from build123d import *

# Parameters (mm, degrees)
CIRPATTERN1_COUNT           = 8
LPATTERN1_START             = -24.818843944
LPATTERN1_OUTLINE_R         = 41.275
LPATTERN1_OUTLINE_R_2       = 38.453474767
LPATTERN1_DEPTH             = 5.187687888
LPATTERN1_START_2           = -12.118843944
LPATTERN1_2_OUTLINE_R       = 41.275
LPATTERN1_2_OUTLINE_R_2     = 38.453474767
LPATTERN1_2_DEPTH           = 5.187687888
SKETCH15_R                  = 53.975
SKETCH15_R_2                = 19.05
BOSS_EXTRUDE1_DEPTH         = 5.08
Q_0_332_DIAMETER_HOLE1_D    = 8.4328
F_1_4_0_25_DIAMETER_HOLE1_D = 6.35
CIRPATTERN2_COUNT           = 6


# Read off the part's stored shape, not the designer's step: LPattern1
with BuildPart() as part:
    # Sketch1 → Revolve1 (revolve)
    with BuildSketch(Plane.XY, mode=Mode.PRIVATE) as revolve1_sk:
        Polygon((-41.275, -40.64), (-41.275, 0), (-34.925, 0), (-34.925, -25.4), (-13.91158, -25.4), (-13.91158, -74.93), (-8.90651, -74.93), (-8.90651, -88.392), (-19.05, -88.392), (-19.05, -40.64), align=None)
    revolve(revolve1_sk.sketch.rotate(Axis((0, 0, 0), (0, 1, 0)), 270), axis=Axis((0, 0, 0), (0, 1, 0)))

    # Sketch8 → 1/4-20 Tapped Hole1 (revolve, cut)
    with BuildSketch(Plane(origin=(38.133127704, -33.02, -15.795258671), x_dir=(-0.38268343236509045, 0, -0.9238795325112865), z_dir=(0, 1, 0))):
        Polygon((0, 0), (0, 14.233816902), (2.5527, 12.7), (2.5527, 0), align=None)
    f_1_4_20_tapped_hole1 = revolve(axis=Axis((43.999762736, -33.02, -18.225298466), (-0.9238795325112865, 0, 0.38268343236509045)), mode=Mode.SUBTRACT)

    # CirPattern1: 1/4-20 Tapped Hole1 ×8 about axis
    cirpattern1_axis = Axis((0, -118.183018713, 0), (0, 1, 0))
    for i in range(1, CIRPATTERN1_COUNT):
        add(f_1_4_20_tapped_hole1.rotate(cirpattern1_axis, i * 360 / CIRPATTERN1_COUNT), mode=Mode.SUBTRACT)

    # LPattern1 outline → LPattern1 (cut)
    with BuildSketch(Plane(origin=(0, 0, 0), x_dir=(1, 0, 0), z_dir=(0, 1, 0)).offset(LPATTERN1_START)):
        Circle(LPATTERN1_OUTLINE_R)
        Circle(LPATTERN1_OUTLINE_R_2, mode=Mode.SUBTRACT)
    extrude(amount=LPATTERN1_DEPTH, mode=Mode.SUBTRACT)

    # LPattern1 2 outline → LPattern1 2 (cut)
    with BuildSketch(Plane(origin=(0, 0, 0), x_dir=(1, 0, 0), z_dir=(0, 1, 0)).offset(LPATTERN1_START_2)):
        Circle(LPATTERN1_2_OUTLINE_R)
        Circle(LPATTERN1_2_OUTLINE_R_2, mode=Mode.SUBTRACT)
    extrude(amount=LPATTERN1_2_DEPTH, mode=Mode.SUBTRACT)

    # Sketch15 → Boss-Extrude1 (add)
    with BuildSketch(Plane.XZ.offset(40.64)):
        with Locations(Location((0, 0, 0), (0, 0, 270))):
            Circle(SKETCH15_R)
        with Locations(Location((0, 0, 0), (0, 0, 270))):
            Circle(SKETCH15_R_2, mode=Mode.SUBTRACT)
    extrude(amount=BOSS_EXTRUDE1_DEPTH)

    # Q (0.332) Diameter Hole1 (through all)
    with Locations(Plane(origin=(0, -45.72, 0), x_dir=(-1, 0, 0), z_dir=(0, -1, 0))):
        with Locations((0, 29.21)):
            Hole(Q_0_332_DIAMETER_HOLE1_D / 2)

    # 1/4 (0.25) Diameter Hole1 (through all)
    with Locations(Plane(origin=(0, -45.72, 0), x_dir=(-1, 0, 0), z_dir=(0, -1, 0))):
        with Locations((0, 49.53)):
            f_1_4_0_25_diameter_hole1 = Hole(F_1_4_0_25_DIAMETER_HOLE1_D / 2)

    # CirPattern2: 1/4 (0.25) Diameter Hole1 ×6 about axis
    cirpattern2_axis = Axis((0, 0, 0), (0, 1, 0))
    for i in range(1, CIRPATTERN2_COUNT):
        add(f_1_4_0_25_diameter_hole1.rotate(cirpattern2_axis, i * 360 / CIRPATTERN2_COUNT), mode=Mode.SUBTRACT)


solid = part.part
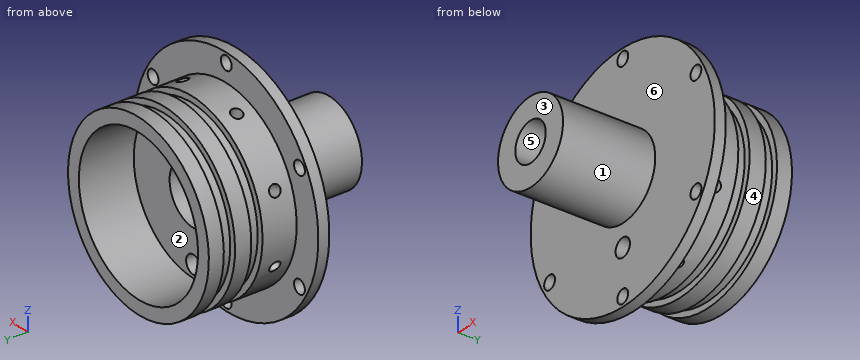
Here's how the part is built. I have some questions about the finished solid (model axes, mm). Face numbers are marked on the shaded views. A direction names the side the tool comes from. Round coordinates to 2 decimals unless told otherwise and drop trailing zeros. Write each loop counter-clockwise with the first axis right and the second up, starting at its lowest first coordinate (ties: lowest second). Pieces come first, ordered by that corner, then holes.
1. Suppose I cut it at A-A (z = 49.53). List the corners of the cut face in (x, y) for me (3 decimals), and give its area (3 significant figures).
2. If we mould it in two halves opening along Z, with no side actions, what happens to the marked faces 1, 2 and 3? For each: released by +Z, released by -Z, zero draft, split by the parting line, or undercut.
3. Will these pins go through, and if not, where does the flat tip stop? pin 1 Ø10 at (x, y) = (-6.5, -76) entering from +Z; pin 2 Ø5 at (x, z) = (-4, -16.5) entering from +Y; pin 3 Ø7.5 at (x, z) = (-42.89, 24.76) entering from -Y; pin 4 Ø2 at (x, y) = (21.5, -76) entering from +Z.
4. Suppose I cut it at D-D (x = -23.5). List the corners of the cut face in (y, z) for me.
5. For the marked faces 4, 5 and 6, which set-ups out of +Z, -Z, +X, -X, +Y, -Y let a thin tool reach every point of the face, with its end or its side?
6. Suppose I cut it at B-B (y = -69). List the corners of the cut face in (x, z) for me.
7. I need wall thicknesses on L1, parallel to Y at x = -31.5, z = 23; L2, parallel to Z at x = 0.5, y = -37; L3, parallel to Y at x = 5.5, z = 32.5. Which ranges of each line are inside material? Lowest first, please.
8. Suppose I cut it at C-C (y = -38). List the corners of the cut face in (x, z) for me (3 decimals), and give its area (3 significant figures).
Answer sheet:
1. outline: (-21.449, -45.72) - (-3.175, -45.72) - (-3.175, -40.64) - (-21.449, -40.64) - close; (3.175, -45.72) - (21.449, -45.72) - (21.449, -40.64) - (3.175, -40.64) - close
1. area: 186 mm2
2. face 1: split by the parting line
2. face 2: undercut
2. face 3: zero draft
3. pin 1: stops at z = 18.99
3. pin 2: stops at y = -25.4
3. pin 3: stops at y = -45.72
3. pin 4: passes through
4. outline: (-45.72, -48.59) - (-40.64, -48.59) - (-40.64, -33.93) - (-24.82, -33.93) - (-24.82, -30.44) - (-19.63, -30.44) - (-19.63, -33.93) - (-12.12, -33.93) - (-12.12, -30.44) - (-6.93, -30.44) - (-6.93, -33.93) - (0, -33.93) - (0, -25.84) - (-25.4, -25.84) - (-25.4, 25.84) - (0, 25.84) - (0, 33.93) - (-6.93, 33.93) - (-6.93, 30.44) - (-12.12, 30.44) - (-12.12, 33.93) - (-19.63, 33.93) - (-19.63, 30.44) - (-24.82, 30.44) - (-24.82, 33.93) - (-40.64, 33.93) - (-40.64, 48.59) - (-45.72, 48.59) - close
5. face 4: +Y
5. face 5: +Y, -Y
5. face 6: -Y
6. outline: circle Ø38.1 at (0, 0); hole circle Ø27.82 at (0, 0)
7. L1: y = -45.72 to -24.82, -19.63 to -12.12, -6.93 to 0
7. L2: z = -41.27 to -33.4, -25.02 to -13.9, 13.9 to 41.27
7. L3: y = -45.72 to -25.4
8. outline: circle Ø82.55 at (0, 0); hole circle Ø27.823 at (0, 0); hole circle Ø8.433 at (0, -29.21)
8. area: 4,690 mm2
